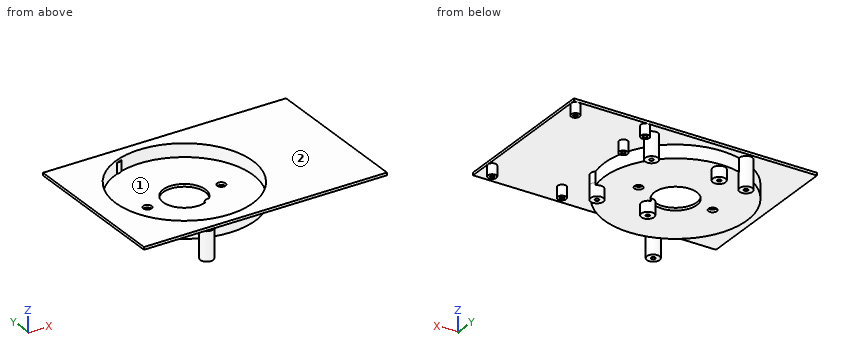
from build123d import *

# Parameters (mm, degrees)
SKETCH1_W                       = 146.05
SKETCH1_H                       = 93.98
SKETCH1_R                       = 41.275
MAIN_DEPTH                      = 1.5875
SKETCH2_R                       = 41.275
SKETCH2_R_2                     = 2.54
SKETCH2_R_3                     = 12.7
DISK_TOP_DEPTH                  = 1.5875
RAISED_START                    = -7.9375
SKETCH3_R                       = 42.8625
SKETCH3_R_2                     = 41.275
RAISED_DISK_DEPTH               = 7.9375
SKETCH4_R                       = 3.81
SKETCH4_R_2                     = 1.2239625
SS_RELAY_MOUNTING_POSTS_DEPTH   = 17.4625
SKETCH5_R                       = 2.54
SKETCH5_R_2                     = 1.190625
MECH_RELAY_MOUNTING_POSTS_DEPTH = 6.35
SKETCH6_R                       = 3.81
SKETCH6_R_2                     = 1.190625
ARDUINO_MOUNTING_1_DEPTH        = 7.9375
SKETCH7_R                       = 3.81
ARDUINO_MOUNTING_2_DEPTH        = 6.35


with BuildPart() as part:
    # Sketch1 → main (new body)
    with BuildSketch(Plane(origin=(0, 0, 7.9375), x_dir=(-1, 0, 0), z_dir=(0, 0, -1))):
        with Locations((-18.415, 0)):
            Rectangle(SKETCH1_W, SKETCH1_H)
        Circle(SKETCH1_R, mode=Mode.SUBTRACT)
    extrude(amount=MAIN_DEPTH)



with BuildPart() as body_2:
    # Sketch2 → disk top (new body)
    with BuildSketch(Plane(origin=(0, 0, 0), x_dir=(-1, 0, 0), z_dir=(0, 0, -1))):
        Circle(SKETCH2_R)
        with Locations((22.225, 0)):
            Circle(SKETCH2_R_2, mode=Mode.SUBTRACT)
        with Locations((-22.225, 0)):
            Circle(SKETCH2_R_2, mode=Mode.SUBTRACT)
        Circle(SKETCH2_R_3, mode=Mode.SUBTRACT)
    extrude(amount=DISK_TOP_DEPTH)


with BuildPart() as part_1:
    add(part.part)

    add(body_2.part)  # raised disk merges body 2
    # Sketch3 → raised disk (add)
    with BuildSketch(Plane(origin=(0, 0, -1.5875), x_dir=(-1, 0, 0), z_dir=(0, 0, -1)).offset(RAISED_START)):
        Circle(SKETCH3_R)
        Circle(SKETCH3_R_2, mode=Mode.SUBTRACT)
    extrude(amount=RAISED_DISK_DEPTH)

    # Sketch4 → SS relay mounting posts (add)
    with BuildSketch(Plane(origin=(0, 0, 6.35), x_dir=(-1, 0, 0), z_dir=(0, 0, -1))):
        with Locations((15.24, 41.91)):
            Circle(SKETCH4_R)
        with Locations((15.24, 41.91)):
            Circle(SKETCH4_R_2, mode=Mode.SUBTRACT)
        with Locations((15.24, -44.45)):
            Circle(SKETCH4_R)
        with Locations((15.24, -44.45)):
            Circle(SKETCH4_R_2, mode=Mode.SUBTRACT)
    extrude(amount=SS_RELAY_MOUNTING_POSTS_DEPTH)

    # Sketch5 → mech relay mounting posts (add)
    with BuildSketch(Plane(origin=(0, 0, 6.35), x_dir=(-1, 0, 0), z_dir=(0, 0, -1))):
        with Locations((-46.99, 44.45)):
            Circle(SKETCH5_R)
        with Locations((-46.99, 44.45)):
            Circle(SKETCH5_R_2, mode=Mode.SUBTRACT)
        with Locations((-88.9, 44.45)):
            Circle(SKETCH5_R)
        with Locations((-88.9, 44.45)):
            Circle(SKETCH5_R_2, mode=Mode.SUBTRACT)
        with Locations((-46.99, 24.13)):
            Circle(SKETCH5_R)
        with Locations((-46.99, 24.13)):
            Circle(SKETCH5_R_2, mode=Mode.SUBTRACT)
        with Locations((-46.99, -33.02)):
            Circle(SKETCH5_R)
        with Locations((-46.99, -33.02)):
            Circle(SKETCH5_R_2, mode=Mode.SUBTRACT)
        with Locations((-88.9, -33.02)):
            Circle(SKETCH5_R)
        with Locations((-88.9, -33.02)):
            Circle(SKETCH5_R_2, mode=Mode.SUBTRACT)
    extrude(amount=MECH_RELAY_MOUNTING_POSTS_DEPTH)

    # Sketch6 → Arduino mounting 1 (add)
    with BuildSketch(Plane.XY.offset(-7.9375)):
        with Locations((39.0525, 38.1)):
            Circle(SKETCH6_R)
        with Locations((39.0525, 38.1)):
            Circle(SKETCH6_R_2, mode=Mode.SUBTRACT)
        with Locations((-1.5875, 38.1)):
            Circle(SKETCH6_R)
        with Locations((-1.5875, 38.1)):
            Circle(SKETCH6_R_2, mode=Mode.SUBTRACT)
        with Locations((8.5725, -12.7)):
            Circle(SKETCH6_R)
        with Locations((8.5725, -12.7)):
            Circle(SKETCH6_R_2, mode=Mode.SUBTRACT)
        with Locations((39.0525, -12.7)):
            Circle(SKETCH6_R)
        with Locations((39.0525, -12.7)):
            Circle(SKETCH6_R_2, mode=Mode.SUBTRACT)
    extrude(amount=ARDUINO_MOUNTING_1_DEPTH)

    # Sketch7 → Arduino mounting 2 (add)
    with BuildSketch(Plane(origin=(0, 0, 6.35), x_dir=(-1, 0, 0), z_dir=(0, 0, -1))):
        with Locations((-39.0525, 38.1)):
            Circle(SKETCH7_R)
        with BuildLine():
            Line((-39.569913642, -16.474703051), (-41.691221214, -9.951682268))
            ThreePointArc((-41.691221214, -9.951682268), (-42.675723267, -13.878283989), (-39.569913642, -16.474703051))
        make_face()
    extrude(amount=ARDUINO_MOUNTING_2_DEPTH)


solid = part_1.part
The model under review builds one solid part; all positions refer to its coordinate system, in mm. Face numbers are marked on the shaded views. Round coordinates to 2 decimals unless told otherwise and drop trailing zeros. Write each loop counter-clockwise with the first axis right and the second up, starting at its lowest first coordinate (ties: lowest second). Pieces come first, ordered by that corner, then holes. Notation, with made-up numbers: (24, 4) -> (48, 4) arc R35 ccw to (48, 43) -> close; hole circle Ø1 at (31, 46). An arc over 180 degrees is marked (long way). Answer as a JSON object with one key per item and string values.
1. The part is to be moulded in two halves that separate along X. For the marked faces 1 and 2, say which applies: pulls with the +X half, pulls with the -X half, needs draft (parallel to the pull), parting line crosses it, or undercut.
Results found:
{"face 1": "undercut", "face 2": "needs draft"}
2. We need section B-B on y = 6. State the section outline as (x, z) points, and give its area (3 significant figures).
Results found:
{"outline": "(-54.61, 6.35) -> (-42.44, 6.35) -> (-42.44, -1.59) -> (-11.19, -1.59) -> (-11.19, 0) -> (-40.84, 0) -> (-40.84, 7.94) -> (-54.61, 7.94) -> close; (11.19, -1.59) -> (42.44, -1.59) -> (42.44, 6.35) -> (91.44, 6.35) -> (91.44, 7.94) -> (40.84, 7.94) -> (40.84, 0) -> (11.19, 0) -> close", "area": "222 mm^2"}
3. To check wall thickness, follow line 1 along X through (y, z) = (-0.5, -1.25); line 2 along Z through (x, y) = (-31, 25); line 3 along Z through (x, y) = (82.5, 15). State the ranges of each line that lie inside material, in increasing order.
Results found:
{"line 1": "x = -42.86 to -24.72, -19.73 to -12.69, 12.69 to 19.73, 24.72 to 42.86", "line 2": "z = -1.59 to 0", "line 3": "z = 6.35 to 7.94"}
4. We need section A-A on z = -4. State how many separate pieces and enclosed holes the cut face has, and give its area (3 significant figures).
Results found:
{"separate pieces": "6", "enclosed holes": "6", "area": "246 mm^2"}
5. We need section D-D on y = -38.5. State the section outline as (x, z) points.
Results found:
{"outline": "(-54.61, 6.35) -> (-18.84, 6.35) -> (-18.84, -1.59) -> (18.84, -1.59) -> (18.84, 6.35) -> (91.44, 6.35) -> (91.44, 7.94) -> (14.88, 7.94) -> (14.88, 0) -> (-14.88, 0) -> (-14.88, 7.94) -> (-54.61, 7.94) -> close"}
6. We need section C-C on y = -19.5. State the section outline as (x, z) points.
Results found:
{"outline": "(-54.61, 6.35) -> (-38.17, 6.35) -> (-38.17, -1.59) -> (38.17, -1.59) -> (38.17, 6.35) -> (91.44, 6.35) -> (91.44, 7.94) -> (36.38, 7.94) -> (36.38, 0) -> (-36.38, 0) -> (-36.38, 7.94) -> (-54.61, 7.94) -> close"}
7. Clearance check with flat-ended pins moving along their axes: pin 1 (1.9 mm diameter, centred on x = -1.59, y = 38.1, fed in from -Z); pin 2 (12 mm diameter, centred on x = -7.5, y = 28.5, fed in from +Z); pin 3 (1.2 mm diameter, centred on x = 89, y = -33, fed in from -Z). State where each tip first meets the part, or that it passes through.
Results found:
{"pin 1": "stops at z = -1.59", "pin 2": "stops at z = 0", "pin 3": "stops at z = 6.35"}
